Design review of the part built by this model. Coordinates are the model's own, in mm. A direction names the side the tool comes from. Give positions to 0.01 mm unless a question says otherwise; leave off trailing zeros. Write each loop counter-clockwise with the first axis right and the second up, starting at its lowest first coordinate (ties: lowest second). Pieces come first, ordered by that corner, then holes. Notation, with made-up numbers: M 46,50.25 L 68,50.25 A25 ccw 68,62.25 Z; hole C 29,44 d5. An arc over 180 degrees is marked long. One line per item, written item: value. Start each with the question number.
```python
from build123d import *

# Parameters (mm, degrees)
F0_W     = 140
F0_H     = 200
F1_DEPTH = 50
F2_W     = 120
F2_H     = 175
F3_DEPTH = 22.5
F4_W     = 120
F4_H     = 175
F5_DEPTH = 22.5
F6_R     = 5


with BuildPart() as f1:
    # F0 (on Front) → F1 (new body)
    with BuildSketch(Plane.XZ):
        with Locations((70, 100)):
            Rectangle(F0_W, F0_H)
    extrude(amount=F1_DEPTH)

    # F2 (on face) → F3 (cut)
    with BuildSketch(Plane.XZ.offset(50)):
        with Locations((70, 100)):
            Rectangle(F2_W, F2_H)
    extrude(amount=-F3_DEPTH, mode=Mode.SUBTRACT)

    # F4 (on face) → F5 (cut)
    with BuildSketch(Plane(origin=(0, 0, 0), x_dir=(-1, 0, 0), z_dir=(0, 1, 0))):
        with Locations((-70, 100)):
            Rectangle(F4_W, F4_H)
    extrude(amount=-F5_DEPTH, mode=Mode.SUBTRACT)

    # F6
    f6_edges = [f1.edges().sort_by_distance(p)[0] for p in [
        (130, -38.75, 187.5),
        (10, -38.75, 187.5),
        (10, -38.75, 12.5),
        (130, -38.75, 12.5),
        (130, -11.25, 187.5),
        (10, -11.25, 187.5),
        (10, -11.25, 12.5),
        (130, -11.25, 12.5),
    ]]
    fillet(f6_edges, radius=F6_R)


solid = f1.part
```
Q1. Wall thickness on line 1 (X direction, y = -12.5, z = 168); line 2 (Z direction, x = 88, y = -18.5); line 3 (Y direction, x = 30, z = 36): over which ranges is each line inside the solid? List them lowest first. Write a range as from..to.
Q2. Take a section at A-A, the plane y = -13.5. Give the boundary of the cut face in (x, z), then the cut area to 3 significant figures.
Q3. Take a section at B-B, the plane x = 49. Give the boundary of the cut face in (y, z), then the cut area to 4 significant figures.
Q4. Take a section at C-C, the plane z = 132.5. Give the boundary of the cut face in (x, y), then the cut area to 3 significant figures.
Q5. For P1, Ø4, axis at x = 97.5, z = 76, coming from the -Y side, flat-tipped, find the tip position at first contact; note if it passes through.
Q6. The part is to be moulded in two halves that separate along X. For faces 1 (the face through (0, -25, 99)), 2 (the face through (11.5, -38.59, 186.07)), 3 (the face through (140, -25, 99)), say which applies: pulls with the +X half, pulls with the -X half, needs draft (parallel to the pull), parting line crosses it, or undercut.
Q7. Machinability: for faces 4 (the face through (128.57, -11.41, 186)), 5 (the face through (69, -39, 187.5)), 6 (the face through (69, -25, 0)), which of the approach directions +Z, -Z, +X, -X, +Y, -Y give a long, thin tool a straight path to every point of the face, cutting with its end or side? Answer none if there is none.
Results list:
1. line 1: x = 0..10, 130..140
1. line 2: z = 0..12.5, 187.5..200
1. line 3: y = -27.5..-22.5
2. outline: M 0,0 L 140,0 L 140,200 L 0,200 Z; hole M 10,17.5 A5 ccw 15,12.5 L 125,12.5 A5 ccw 130,17.5 L 130,182.5 A5 ccw 125,187.5 L 15,187.5 A5 ccw 10,182.5 Z
2. area: 7,020 mm^2
3. outline: M -50,0 L 0,0 L 0,12.5 L -22.5,12.5 L -22.5,187.5 L 0,187.5 L 0,200 L -50,200 L -50,187.5 L -27.5,187.5 L -27.5,12.5 L -50,12.5 Z
3. area: 2,125 mm^2
4. outline: M 0,-50 L 10,-50 L 10,-27.5 L 130,-27.5 L 130,-50 L 140,-50 L 140,0 L 130,0 L 130,-22.5 L 10,-22.5 L 10,0 L 0,0 Z
4. area: 1,600 mm^2
5. P1: stops at y = -27.5
6. face 1: pulls with the -X half
6. face 2: undercut
6. face 3: pulls with the +X half
7. face 4: +Y
7. face 5: -Y
7. face 6: -Z, +X, -X, +Y, -Y
